Input: part model. Units: mm. Frame: model coordinates. Face numbers are marked on the shaded views. A direction names the side the tool comes from. Coordinates: 2 decimals unless noted, no trailing zeros. Write each loop counter-clockwise with the first axis right and the second up, starting at its lowest first coordinate (ties: lowest second). Pieces come first, ordered by that corner, then holes. Notation, with made-up numbers: (53.5, -24) - (58.5, -24) arc R23 ccw to (58.5, 14) - close; hole circle Ø10 at (-39, 44). An arc over 180 degrees is marked (long way). Use a Markdown table: item, result. Add a question column.
Q1. Section query A-A (z = -1.75). Return the cut outline in (x, y) (3 decimals), then the cut area to 3 significant figures.
Q2. Pin query (flat end, axial travel): P1, Ø5, axis at y = 18.5, z = -12.5, coming from the +X side; P2, Ø4, axis at x = 11.21, y = 27.75, coming from the -Z side; P3, Ø3, axis at y = 1.75, z = -1.75, coming from the -X side; P4, Ø1.8, axis at x = 10.5, z = -3, coming from the -Y side. Return the tip coordinate at first contact, or that it passes through.
Q3. Set-up query: the marked faces 1, 2, 3 and 4. Return all of +Z, -Z, +X, -X, +Y, -Y with unobstructed straight access to the full face (end or side cutting, diameter ignored); none if empty.
Q4. Section query D-D (y = 1.75). Return the cut outline in (x, z) (3 decimals).
Q5. Material intervals for probe 1 along Y at (x, z) = (1.5, -20.69) (3 decimals); probe 2 along Y at (x, z) = (1.6, -11.22); probe 3 along X at (y, z) = (3, -2), sorted ascending. Write a range as from..to.
Q6. Section query C-C (z = -20.69). Return the cut outline in (x, y) (3 decimals).
Q7. Section query B-B (y = 18.5). Return the cut outline in (x, z), then the cut area to 3 significant figures.
from build123d import *

# Parameters (mm, degrees)
BOSS_EXTRUDE1_DEPTH = 37
FILLET1_R           = 3
SKETCH2_R           = 1.5
SKETCH2_W           = 19.44
SKETCH2_H           = 3.5
CUT_EXTRUDE1_DEPTH  = 49.745330033
SKETCH3_R           = 0.975
SKETCH3_R_2         = 2.75
CUT_EXTRUDE2_DEPTH  = 49.745330033


with BuildPart() as part:
    # Sketch1 → Boss-Extrude1 (new body)
    with BuildSketch(Plane(origin=(0, 0, 0), x_dir=(1, 0, 0), z_dir=(0, 1, 0))):
        Polygon((0, 0), (22.44, 0), (22.44, 3), (3, 3), (3, 22.44), (0, 22.44), align=None)
    extrude(amount=BOSS_EXTRUDE1_DEPTH)

    # Fillet1
    fillet1_edges = [part.edges().sort_by_distance(p)[0] for p in [
        (3, 18.5, -3),
    ]]
    fillet(fillet1_edges, radius=FILLET1_R)

    # Sketch2 → Cut-Extrude1 (cut, through all)
    with BuildSketch(Plane(origin=(0, 0, -22.44), x_dir=(-1, 0, 0), z_dir=(0, 0, -1))):
        with Locations((-11.212785563, 27.75)):
            Circle(SKETCH2_R)
        with Locations((-17.212785563, 18.5)):
            Circle(SKETCH2_R)
        with Locations((-11.212785563, 9.25)):
            Circle(SKETCH2_R)
        with Locations((-12.72, 1.75)):
            Rectangle(SKETCH2_W, SKETCH2_H)
        with Locations((-12.72, 35.25)):
            Rectangle(SKETCH2_W, SKETCH2_H)
    extrude(amount=-CUT_EXTRUDE1_DEPTH, mode=Mode.SUBTRACT)

    # Sketch3 → Cut-Extrude2 (cut, through all)
    with BuildSketch(Plane.ZY):
        with Locations((-1.75, 35.25)):
            Circle(SKETCH3_R)
        with Locations((-1.75, 1.75)):
            Circle(SKETCH3_R)
        with Locations((-20.69, 1.75)):
            Circle(SKETCH3_R)
        with Locations((-20.69, 35.25)):
            Circle(SKETCH3_R)
        with Locations((-11.22, 26)):
            Circle(SKETCH3_R_2)
    extrude(amount=-CUT_EXTRUDE2_DEPTH, mode=Mode.SUBTRACT)


solid = part.part
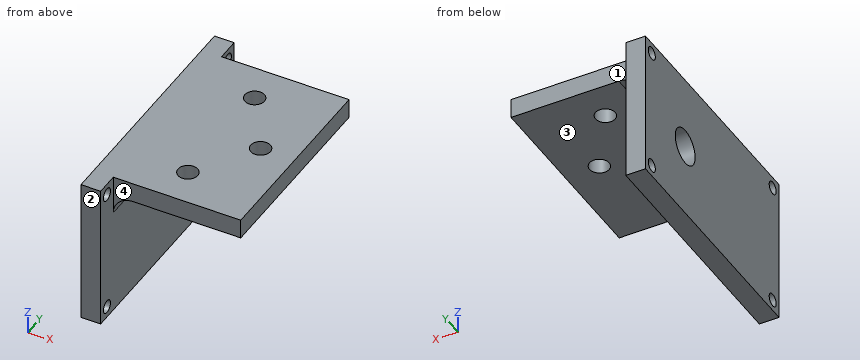
Values follow:
| question | item | result |
|---|---|---|
| 1 | outline | (0, 0) - (3, 0) - (3, 0.775) - (0, 0.775) - close; (0, 2.725) - (3, 2.725) - (3, 3.5) - (22.44, 3.5) - (22.44, 33.5) - (3, 33.5) - (3, 34.275) - (0, 34.275) - close; (0, 36.225) - (3, 36.225) - (3, 37) - (0, 37) - close; hole circle Ø3 at (11.213, 9.25); hole circle Ø3 at (11.213, 27.75); hole circle Ø3 at (17.213, 18.5) |
| 1 | area | 661 mm2 |
| 2 | P1 | x = 3 |
| 2 | P2 | z = -3 |
| 2 | P3 | x = 0 |
| 2 | P4 | y = 3.5 |
| 3 | face 1 | +Z, -Z, +X, +Y |
| 3 | face 2 | +Z, -Z, +X, -X, -Y |
| 3 | face 3 | -Z, +X, +Y, -Y |
| 3 | face 4 | +Z, -Z, +X, -Y |
| 4 | outline | (0, -22.44) - (3, -22.44) - (3, -21.665) - (0, -21.665) - close; (0, -19.715) - (3, -19.715) - (3, -2.725) - (0, -2.725) - close; (0, -0.775) - (3, -0.775) - (3, 0) - (0, 0) - close |
| 5 | probe 1 | 0..0.775, 2.725..34.275, 36.225..37 |
| 5 | probe 2 | 0..23.25, 28.75..37 |
| 5 | probe 3 | 0..3 |
| 6 | outline | (0, 0) - (3, 0) - (3, 0.775) - (0, 0.775) - close; (0, 2.725) - (3, 2.725) - (3, 34.275) - (0, 34.275) - close; (0, 36.225) - (3, 36.225) - (3, 37) - (0, 37) - close |
| 7 | outline | (0, -22.44) - (3, -22.44) - (3, -6) arc R3 cw to (6, -3) - (15.71, -3) - (15.71, 0) - (0, 0) - close; (18.71, -3) - (22.44, -3) - (22.44, 0) - (18.71, 0) - close |
| 7 | area | 119 mm2 |
